```python
from build123d import *

# Parameters (mm, degrees)
SKETCH1_R           = 12.000000003
BOSS_EXTRUDE1_DEPTH = 13
SKETCH2_R           = 12.000000003
CUT_EXTRUDE1_DEPTH  = 6
BOSS_EXTRUDE2_START = -1.5
SKETCH3_R           = 12.000000003
SKETCH3_R_2         = 8
BOSS_EXTRUDE2_DEPTH = 1.5
SKETCH4_W           = 40.64
SKETCH4_H           = 6
CUT_EXTRUDE2_DEPTH  = 107.967410462
BOSS_EXTRUDE3_START = 5.499999908
SKETCH6_R           = 12.000000003
SKETCH6_R_2         = 10.5
BOSS_EXTRUDE3_DEPTH = 5.499999908
MOVE_FACE3_BY       = 1.000000032


with BuildPart() as part:
    # Sketch1 → Boss-Extrude1 (new body)
    with BuildSketch(Plane(origin=(0, 0, 0), x_dir=(1, 0, 0), z_dir=(0, 1, 0))):
        with BuildLine():
            Line((-18.350000003, 0), (-18.350000003, 81.28))
            ThreePointArc((-18.350000003, 81.28), (0, 99.630000003), (18.350000003, 81.28))
            Line((18.350000003, 81.28), (18.350000003, 0))
            ThreePointArc((18.350000003, 0), (0, -18.350000003), (-18.350000003, 0))
        make_face()
        with Locations(Location((0, 0, 0), (0, 0, 270))):
            Circle(SKETCH1_R, mode=Mode.SUBTRACT)
        with Locations(Location((0, 81.28, 0), (0, 0, 270))):
            Circle(SKETCH1_R, mode=Mode.SUBTRACT)
    extrude(amount=BOSS_EXTRUDE1_DEPTH)

    # Sketch2 → Cut-Extrude1 (cut)
    # profile 1 of 2: a face of its own
    with BuildSketch(Plane.XZ):
        with BuildLine():
            Line((-18.350000003, -60.96), (-18.350000003, -81.28))
            ThreePointArc((-18.350000003, -81.28), (0, -99.630000003), (18.350000003, -81.28))
            Line((18.350000003, -81.28), (18.350000003, -60.96))
            Line((18.350000003, -60.96), (-18.350000003, -60.96))
        make_face()
        with Locations(Location((0, -81.28, 0), (0, 0, 270))):
            Circle(SKETCH2_R, mode=Mode.SUBTRACT)
    # profile 2 of 2: a face of its own
    with BuildSketch(Plane.XZ):
        with BuildLine():
            ThreePointArc((18.350000003, 0), (0, 18.350000003), (-18.350000003, 0))
            Line((-18.350000003, 0), (-18.350000003, -20.32))
            Line((-18.350000003, -20.32), (18.350000003, -20.32))
            Line((18.350000003, -20.32), (18.350000003, 0))
        make_face()
    extrude(amount=-CUT_EXTRUDE1_DEPTH, mode=Mode.SUBTRACT)

    # Sketch3 → Boss-Extrude2 (add)
    # profile 1 of 2: a face of its own
    with BuildSketch(Plane(origin=(0, 12.999999908, 0), x_dir=(1, 0, 0), z_dir=(0, 1, 0)).offset(BOSS_EXTRUDE2_START)):
        with Locations(Location((0, 81.28, 0), (0, 0, 90))):
            Circle(SKETCH3_R)
        with Locations(Location((0, 81.28, 0), (0, 0, 270))):
            Circle(SKETCH3_R_2, mode=Mode.SUBTRACT)
    # profile 2 of 2: a face of its own
    with BuildSketch(Plane(origin=(0, 12.999999908, 0), x_dir=(1, 0, 0), z_dir=(0, 1, 0)).offset(BOSS_EXTRUDE2_START)):
        with Locations(Location((0, 0, 0), (0, 0, 90))):
            Circle(SKETCH3_R)
        with Locations(Location((0, 0, 0), (0, 0, 270))):
            Circle(SKETCH3_R_2, mode=Mode.SUBTRACT)
    extrude(amount=BOSS_EXTRUDE2_DEPTH)

    # Sketch4 → Cut-Extrude2 (cut, through all)
    with BuildSketch(Plane.ZY.offset(18.350000003)):
        with Locations((-40.64, 3)):
            Rectangle(SKETCH4_W, SKETCH4_H)
    extrude(amount=-CUT_EXTRUDE2_DEPTH, mode=Mode.SUBTRACT)

    # Sketch6 → Boss-Extrude3 (add)
    with BuildSketch(Plane.XZ.offset(-11.499999908).offset(BOSS_EXTRUDE3_START)):
        Circle(SKETCH6_R)
        with Locations(Location((0, 0, 0), (0, 0, 270))):
            Circle(SKETCH6_R_2, mode=Mode.SUBTRACT)
    extrude(amount=-BOSS_EXTRUDE3_DEPTH)

    # Move Face3: a face moved outward by 1.0
    extrude(part.faces().sort_by_distance((0, 11.499999908, 8.4))[0], amount=MOVE_FACE3_BY, dir=(0, -1, 0))


solid = part.part
```
CAD build for the part. Positions are in the model's coordinates, mm. A direction names the side the tool comes from. Round coordinates to 2 decimals unless told otherwise and drop trailing zeros. Order: outer loops, then holes, each group sorted by start corner. A loop starts at its lowest first (then second) coordinate and runs counter-clockwise, first axis right, second up. Notation, with made-up numbers: (-14, -28.5) - (22, -28.5) arc R23 cw to (22, 8.5) - close; hole circle Ø2 at (40.25, 19.5). An arc over 180 degrees is marked (long way). Answer in a Markdown table with one row per item. Add a question column.
(1) Mould opens along Z. For faces 1 (the face through (0.352, 12.239, -89.272)), 2 (the face through (-18.35, 9, -40)), 3 (the face through (3.2, 8.2, -10)), 4 (the face through (0.404, 9.451, 18.346)) say: +Z half, -Z half, draft (parallel to the pull), parting line (faces both ways), or undercut.
(2) Band-saw the part on B-B on y = 9. List the corners of the cut face in (x, z).
(3) Band-saw the part on D-D on x = -14. List the corners of the cut face in (y, z), and give its area (3 significant figures).
(4) 3-axis set-ups, long thin cutter, end or side, ignore diameter. For faces 5 (the face through (3.604, 8.711, -69.834)), 6 (the face through (18.35, 9, -41)): which of +Z, -Z, +X, -X, +Y, -Y reach the whole face in a straight line?
(5) Band-saw the part on A-A on x = 0. List the corners of the cut face in (y, z).
(6) Probe L1, parallel to Z at x = -8.5, y = 8.5; L2, parallel to X at y = 12.3, z = -81.28; L3, parallel to Z at x = 3, y = 11. List the from-to ranges inside material, lowest first. Write a range as [from, to].
(7) Band-saw the part on C-C on x = 5.5. List the corners of the cut face in (y, z), and give its area (3 significant figures).
(8) Drop flat-ended pins along their axis: pin 1 Ø1 at (x, y) = (8, 10.5) entering from +Z; pin 2 Ø17 at (x, z) = (0, 0) entering from -Y. Give the stop position or say it passes through.
Data:
| question | item | result |
|---|---|---|
| 1 | face 1 | undercut |
| 1 | face 2 | draft |
| 1 | face 3 | undercut |
| 1 | face 4 | +Z half |
| 2 | outline | (-18.35, -81.28) arc R18.35 ccw to (18.35, -81.28) - (18.35, 0) arc R18.35 ccw to (-18.35, 0) - close; hole circle Ø24 at (0, -81.28); hole circle Ø21 at (0, 0) |
| 3 | outline | (6, -93.14) - (13, -93.14) - (13, 11.86) - (6, 11.86) - close |
| 3 | area | 735 mm^2 |
| 4 | face 5 | -Y |
| 4 | face 6 | +Z, -Z, +X, +Y, -Y |
| 5 | outline | (6, -99.63) - (13, -99.63) - (13, -89.28) - (11.5, -89.28) - (11.5, -93.28) - (6, -93.28) - close; (6, -69.28) - (11.5, -69.28) - (11.5, -73.28) - (13, -73.28) - (13, -8) - (10.5, -8) - (10.5, -10.5) - (6, -10.5) - close; (6, 10.5) - (10.5, 10.5) - (10.5, 8) - (13, 8) - (13, 18.35) - (6, 18.35) - close |
| 6 | L1 | z = [-97.54, -89.75], [-72.81, -6.16], [6.16, 16.26] |
| 6 | L2 | x = [-18.35, -8], [8, 18.35] |
| 6 | L3 | z = [-99.38, -92.9], [-69.66, -7.42], [7.42, 18.1] |
| 7 | outline | (6, -98.79) - (13, -98.79) - (13, -87.09) - (11.5, -87.09) - (11.5, -91.95) - (6, -91.95) - close; (6, -70.61) - (11.5, -70.61) - (11.5, -75.47) - (13, -75.47) - (13, -5.81) - (10.5, -5.81) - (10.5, -8.94) - (6, -8.94) - close; (6, 8.94) - (10.5, 8.94) - (10.5, 5.81) - (13, 5.81) - (13, 17.51) - (6, 17.51) - close |
| 7 | area | 570 mm^2 |
| 8 | pin 1 | stops at z = 16.75 |
| 8 | pin 2 | stops at y = 10.5 |
